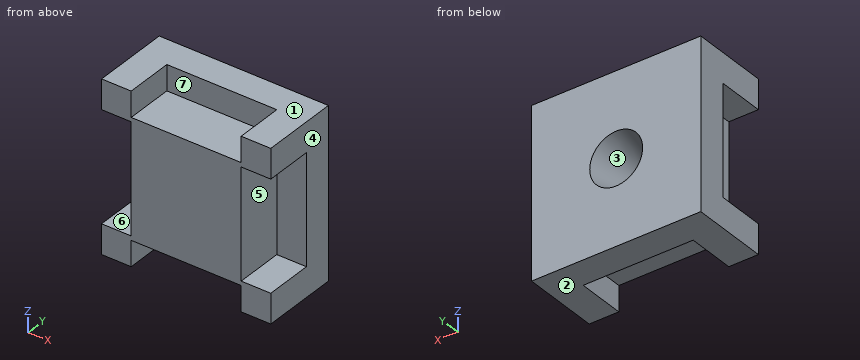
```python
from build123d import *

# Parameters (mm, degrees)
ESBO_O1_W                  = 40
ESBO_O1_H                  = 40
RESSALTO_EXTRUS_O1_DEPTH   = 40
ESBO_O10_W                 = 26
ESBO_O10_H                 = 26
CORTE_EXTRUS_O3_DEPTH      = 7
ESBO_O11_W                 = 26
ESBO_O11_H                 = 26
CORTE_EXTRUS_O6_DEPTH      = 6
ESBO_O12_W                 = 26
ESBO_O12_H                 = 26
CORTE_EXTRUS_O7_DEPTH      = 6
ESBO_O13_W                 = 26
ESBO_O13_H                 = 26
CORTE_EXTRUS_O8_DEPTH      = 7
ESBO_O2_R                  = 6.255
ESBO_O4_R                  = 2.41
FILETE2_R                  = 0.5
CORTE_EXTRUS_O9_DEPTH      = 37
CORTE_EXTRUS_O9_DEPTH_BACK = 37
ESBO_O14_W                 = 40
ESBO_O14_H                 = 21.655550529


with BuildPart() as part:
    # Esboço1 → Ressalto-extrusão1 (new body)
    with BuildSketch(Plane(origin=(0, 0, 0), x_dir=(1, 0, 0), z_dir=(0, 1, 0))):
        with Locations((-13.703200382, -28.10068404)):
            Rectangle(ESBO_O1_W, ESBO_O1_H)
    extrude(amount=RESSALTO_EXTRUS_O1_DEPTH)

    # Esboço10 → Corte-extrusão3 (cut)
    with BuildSketch(Plane.ZY.offset(33.703200382)):
        with Locations((28.10068404, 20)):
            Rectangle(ESBO_O10_W, ESBO_O10_H)
    extrude(amount=-CORTE_EXTRUS_O3_DEPTH, mode=Mode.SUBTRACT)

    # Esboço11 → Corte-extrusão6 (cut)
    with BuildSketch(Plane(origin=(0, 0, 8.10068404), x_dir=(-1, 0, 0), z_dir=(0, 0, -1))):
        with Locations((13.703200382, 20)):
            Rectangle(ESBO_O11_W, ESBO_O11_H)
    extrude(amount=-CORTE_EXTRUS_O6_DEPTH, mode=Mode.SUBTRACT)

    # Esboço12 → Corte-extrusão7 (cut)
    with BuildSketch(Plane.XY.offset(48.10068404)):
        with Locations((-13.703200382, 20)):
            Rectangle(ESBO_O12_W, ESBO_O12_H)
    extrude(amount=-CORTE_EXTRUS_O7_DEPTH, mode=Mode.SUBTRACT)

    # Esboço13 → Corte-extrusão8 (cut)
    with BuildSketch(Plane(origin=(6.296799618, 0, 0), x_dir=(0, 0, -1), z_dir=(1, 0, 0))):
        with Locations((-28.10068404, 20)):
            Rectangle(ESBO_O13_W, ESBO_O13_H)
    extrude(amount=-CORTE_EXTRUS_O8_DEPTH, mode=Mode.SUBTRACT)

    # Esboço2 → Loft de corte2 section 0
    with BuildSketch(Plane(origin=(0, 40, 0), x_dir=(1, 0, 0), z_dir=(0, 1, 0))):
        with Locations((-13.703200382, -28.10068404)):
            Circle(ESBO_O2_R)
    # Esboço4 → Loft de corte2 section 1
    with BuildSketch(Plane(origin=(0, 24.13, 0), x_dir=(1, 0, 0), z_dir=(0, 1, 0))):
        with Locations((-13.703200382, -28.10068404)):
            Circle(ESBO_O4_R)
    loft(mode=Mode.SUBTRACT)

    # Filete2
    filete2_edges = [part.edges().sort_by_distance(p)[0] for p in [
        (-16.113200382, 24.13, 28.10068404),
    ]]
    fillet(filete2_edges, radius=FILETE2_R)

    # Esboço14 → Corte-extrusão9 (cut, two sides: drawn at the far end of the back side and taken through both)
    with BuildSketch(Plane(origin=(0, 0, 14.10068404), x_dir=(-1, 0, 0), z_dir=(0, 0, -1)).offset(-CORTE_EXTRUS_O9_DEPTH_BACK)):
        with Locations((13.703200382, 10.827775265)):
            Rectangle(ESBO_O14_W, ESBO_O14_H)
    extrude(amount=CORTE_EXTRUS_O9_DEPTH + CORTE_EXTRUS_O9_DEPTH_BACK, mode=Mode.SUBTRACT)


solid = part.part
```
Build history of the part. All positions in model axes, mm. Face numbers are marked on the shaded views. A direction names the side the tool comes from. Give positions to 0.01 mm unless a question says otherwise; leave off trailing zeros. Loops run counter-clockwise (first coordinate to the right, second up) from the corner with the lowest first, then second, coordinate; pieces in that order, holes last.
Item 1: Slice it at A-A, the plane x = -24.5. List the corners of the cut face in (y, z), and give its area (3 significant figures).
Answers follow:
outline: (21.66, 14.1) - (33, 14.1) - (33, 8.1) - (40, 8.1) - (40, 48.1) - (33, 48.1) - (33, 42.1) - (21.66, 42.1) - close
area: 598 mm2
Item 2: Flat gauge pins, fed straight in: pin 1 (5.5 mm diameter, centred on x = -20, y = 25.5, fed in from +Z); pin 2 (9 mm diameter, centred on y = 26.5, z = 23.5, fed in from -X); pin 3 (3.5 mm diameter, centred on x = 1.5, z = 28.5, fed in from -Y). Where does each tip first touch, or does it go through?
Answers follow:
pin 1: stops at z = 42.1
pin 2: stops at x = -26.7
pin 3: stops at y = 33
Item 3: Slice it at D-D, the plane z = 43. List the corners of the cut face in (x, y).
Answers follow:
outline: (-33.7, 21.66) - (-26.7, 21.66) - (-26.7, 33) - (-0.7, 33) - (-0.7, 21.66) - (6.3, 21.66) - (6.3, 40) - (-33.7, 40) - close
Item 4: Pull direction Z, two halves, no side cores. Call the marked faces 1, 2, 3 and 4: released by +Z, released by -Z, zero draft, split by the parting line, or undercut.
Answers follow:
face 1: released by +Z
face 2: released by -Z
face 3: undercut
face 4: zero draft
Item 5: Slice it at C-C, the plane y = 30.25. List the corners of the cut face in (x, z), and give its area (3 significant figures).
Answers follow:
outline: (-33.7, 8.1) - (-26.7, 8.1) - (-26.7, 14.1) - (-0.7, 14.1) - (-0.7, 8.1) - (6.3, 8.1) - (6.3, 15.1) - (-0.7, 15.1) - (-0.7, 41.1) - (6.3, 41.1) - (6.3, 48.1) - (-0.7, 48.1) - (-0.7, 42.1) - (-26.7, 42.1) - (-26.7, 48.1) - (-33.7, 48.1) - (-33.7, 41.1) - (-26.7, 41.1) - (-26.7, 15.1) - (-33.7, 15.1) - close; hole circle Ø7.79 at (-13.7, 28.1)
area: 876 mm2
Item 6: Drill centre lines: line 1 (Z direction, x = 2.5, y = 27.5); line 2 (X direction, y = 24.75, z = 44.5); line 3 (X direction, y = 24, z = 20). Where is each one in solid material? Low to high.
Answers follow:
line 1: z = 8.1 to 15.1, 41.1 to 48.1
line 2: x = -33.7 to -26.7, -0.7 to 6.3
line 3: x = -26.7 to -0.7
Item 7: Slice it at B-B, the plane y = 23.25. List the corners of the cut face in (x, z), and give its area (3 significant figures).
Answers follow:
outline: (-33.7, 8.1) - (-26.7, 8.1) - (-26.7, 14.1) - (-0.7, 14.1) - (-0.7, 8.1) - (6.3, 8.1) - (6.3, 15.1) - (-0.7, 15.1) - (-0.7, 41.1) - (6.3, 41.1) - (6.3, 48.1) - (-0.7, 48.1) - (-0.7, 42.1) - (-26.7, 42.1) - (-26.7, 48.1) - (-33.7, 48.1) - (-33.7, 41.1) - (-26.7, 41.1) - (-26.7, 15.1) - (-33.7, 15.1) - close
area: 924 mm2
Item 8: Which spindle directions (+Z, -Z, +X, -X, +Y, -Y) get a long thin tool onto all of the face, cutting with end or side? Do the marked faces 5, 6 and 7. Say none if no direction does.
Answers follow:
face 5: +X, -Y
face 6: -X, -Y
face 7: +Z, -Y
